Geometry: see drawing. Coordinates: mm, zero at the bounding-box minimum. A direction names the side the tool comes from. Give positions to 0.01 mm unless a question says otherwise; leave off trailing zeros. Write each loop counter-clockwise with the first axis right and the second up, starting at its lowest first coordinate (ties: lowest second). Pieces come first, ordered by that corner, then holes. Notation, with made-up numbers: M 34.5,59 L 39.5,59 A20 ccw 39.5,85 Z; hole C 51,74.5 d6. An arc over 180 degrees is marked long. Use a Markdown table: item, result. Add a question column.
1) Set-up query: the marked faces 1 and 2. Return all of +Z, -Z, +X, -X, +Y, -Y with unobstructed straight access to the full face (end or side cutting, diameter ignored); none if empty.
2) Section A-A on y = 1096. Return the cut outline in (x, z).
3) Draft query along Z for the marked faces 3, 4, 5 and 6. Return one class per face: +Z half, -Z half, draft (parallel to the pull), parting line (faces both ways), or undercut.
4) Section B-B on z = 42. Return the cut outline in (x, y), then the cut area to 3 significant figures.
5) Section D-D on x = 560. State how many separate pieces and enclosed holes the cut face has, then the cut area to 3 significant figures.
6) Section C-C on y = 487. Return the cut outline in (x, z), then the cut area to 3 significant figures.
7) Pin query (flat end, axial travel): pin 1 (15 mm diameter, centred on x = 1189.5, y = 362, fed in from -Z). Return the tip coordinate at first contact, or that it passes through.
8) Line query: line 1 (Y direction, x = 1017.5, z = 9); line 2 (X direction, y = 276.5, z = 123); line 3 (Z direction, x = 799.5, y = 251). Output: solid intervals per line, ascending.
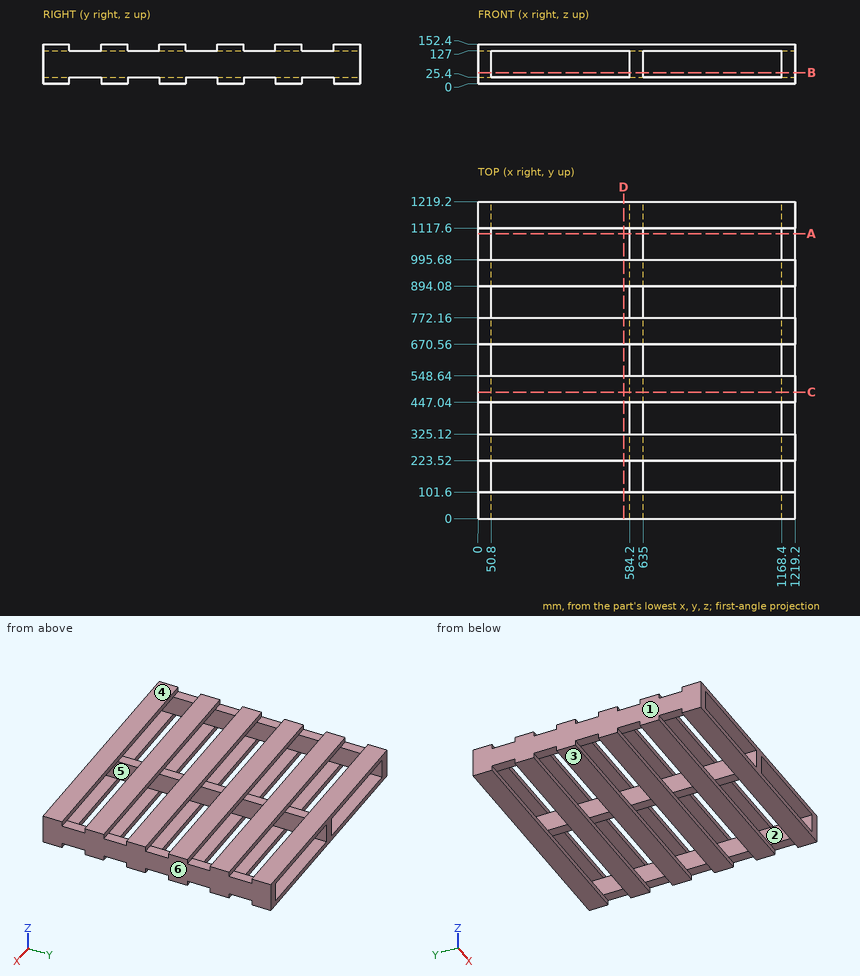
Found:
| question | item | result |
|---|---|---|
| 1 | face 1 | +Z, -Z, -X, +Y, -Y |
| 1 | face 2 | +Y, -Y |
| 2 | outline | M 0,25.4 L 50.8,25.4 L 50.8,127 L 0,127 Z; M 584.2,25.4 L 635,25.4 L 635,127 L 584.2,127 Z; M 1168.4,25.4 L 1219.2,25.4 L 1219.2,127 L 1168.4,127 Z |
| 3 | face 3 | -Z half |
| 3 | face 4 | +Z half |
| 3 | face 5 | undercut |
| 3 | face 6 | draft |
| 4 | outline | M 0,0 L 50.8,0 L 50.8,1219.2 L 0,1219.2 Z; M 584.2,0 L 635,0 L 635,1219.2 L 584.2,1219.2 Z; M 1168.4,0 L 1219.2,0 L 1219.2,1219.2 L 1168.4,1219.2 Z |
| 4 | area | 186,000 mm² |
| 5 | separate pieces | 12 |
| 5 | enclosed holes | 0 |
| 5 | area | 31,000 mm² |
| 6 | outline | M 0,0 L 1219.2,0 L 1219.2,152.4 L 0,152.4 Z; hole M 50.8,25.4 L 584.2,25.4 L 584.2,127 L 50.8,127 Z; hole M 635,25.4 L 1168.4,25.4 L 1168.4,127 L 635,127 Z |
| 6 | area | 77,400 mm² |
| 7 | pin 1 | z = 25.4 |
| 8 | line 1 | 0 to 101.6, 223.52 to 325.12, 447.04 to 548.64, 670.56 to 772.16, 894.08 to 995.68, 1117.6 to 1219.2 |
| 8 | line 2 | 0 to 50.8, 584.2 to 635, 1168.4 to 1219.2 |
| 8 | line 3 | 0 to 25.4, 127 to 152.4 |
